Build history of the part. All positions in model axes, mm. A direction names the side the tool comes from. Give positions to 0.01 mm unless a question says otherwise; leave off trailing zeros. Order: outer loops, then holes, each group sorted by start corner. A loop starts at its lowest first (then second) coordinate and runs counter-clockwise, first axis right, second up. Notation, with made-up numbers: (56, 83.25) - (107, 83.25) arc R38 ccw to (107, 122.25) - close; hole circle Ø5 at (-36.5, 85). An arc over 180 degrees is marked (long way). Use a Markdown table: item, result.
from build123d import *

# Parameters (mm, degrees)
BASE_PLATE_DEPTH                        = 4.7625
OUTSIDEBOSS_DEPTH                       = 50.8
TOPPLATE_MOUNTINGHOLE_8_0_199_DIAMETE_D = 5.1054
PCB_PLATE_DEPTH                         = 12.7
F_4_CLEARANCE_HOLE1_D                   = 3.2639
F_4_CLEARANCE_HOLE1_DEPTH               = 16.002
F_4_CLEARANCE_HOLE1_TIP                 = 0.980574487
SKETCH11_W                              = 87.3125
SKETCH11_H                              = 50.8
SKETCH11_W_2                            = 6.35
SKETCH11_H_2                            = 6.35
CUT_EXTRUDE2_DEPTH                      = 4.7625
SKETCH12_W                              = 78.3336
SKETCH12_H                              = 18.0086
SKETCH12_W_2                            = 76.2
SKETCH12_H_2                            = 15.875
BATTERYHOLDER_DEPTH                     = 44.45
BATTERYLEADFEADER_REACH                 = 128.453
BATTERYLEADFILLETS_R                    = 3.175
CUT_EXTRUDE3_REACH                      = 149.637


with BuildPart() as part:
    # Sketch1 → Base_Plate (new body)
    with BuildSketch(Plane(origin=(0, 0, 0), x_dir=(1, 0, 0), z_dir=(0, 1, 0))):
        with BuildLine():
            Line((-53.975, 50.8), (53.975, 50.8))
            ThreePointArc((53.975, 50.8), (60.710192091, 48.010192091), (63.5, 41.275))
            Line((63.5, 41.275), (63.5, -41.275))
            ThreePointArc((63.5, -41.275), (60.710192091, -48.010192091), (53.975, -50.8))
            Line((53.975, -50.8), (-53.975, -50.8))
            ThreePointArc((-53.975, -50.8), (-60.710192091, -48.010192091), (-63.5, -41.275))
            Line((-63.5, -41.275), (-63.5, 41.275))
            ThreePointArc((-63.5, 41.275), (-60.710192091, 48.010192091), (-53.975, 50.8))
        make_face()
    extrude(amount=BASE_PLATE_DEPTH)

    # Sketch2 → OutsideBoss (add)
    with BuildSketch(Plane(origin=(0, 4.7625, 0), x_dir=(1, 0, 0), z_dir=(0, 1, 0))):
        with BuildLine():
            Line((-53.975, -50.8), (53.975, -50.8))
            ThreePointArc((53.975, -50.8), (60.710192091, -48.010192091), (63.5, -41.275))
            Line((63.5, -41.275), (63.5, 41.275))
            ThreePointArc((63.5, 41.275), (60.710192091, 48.010192091), (53.975, 50.8))
            Line((53.975, 50.8), (-53.975, 50.8))
            ThreePointArc((-53.975, 50.8), (-60.710192091, 48.010192091), (-63.5, 41.275))
            Line((-63.5, 41.275), (-63.5, -41.275))
            ThreePointArc((-63.5, -41.275), (-60.710192091, -48.010192091), (-53.975, -50.8))
        make_face()
        with BuildLine():
            Line((-56.1975, 41.275), (-56.1975, -41.275))
            ThreePointArc((-56.1975, -41.275), (-55.546544821, -42.846544821), (-53.975, -43.4975))
            Line((-53.975, -43.4975), (53.975, -43.4975))
            ThreePointArc((53.975, -43.4975), (55.546544821, -42.846544821), (56.1975, -41.275))
            Line((56.1975, -41.275), (56.1975, 41.275))
            ThreePointArc((56.1975, 41.275), (55.546544821, 42.846544821), (53.975, 43.4975))
            Line((53.975, 43.4975), (-53.975, 43.4975))
            ThreePointArc((-53.975, 43.4975), (-55.546544821, 42.846544821), (-56.1975, 41.275))
        make_face(mode=Mode.SUBTRACT)
    extrude(amount=OUTSIDEBOSS_DEPTH)

    # TopPlate_MountingHole_#8 (0.199) Diameter Hole1 (through all)
    with Locations(Plane(origin=(0, 0, 0), x_dir=(-1, 0, 0), z_dir=(0, -1, 0))):
        with Locations((-58.07075, 45.37075), (58.07075, -45.37075), (-58.07075, -45.37075), (58.07075, 45.37075)):
            Hole(TOPPLATE_MOUNTINGHOLE_8_0_199_DIAMETE_D / 2)

    # Sketch8 → PCB_Plate (add)
    with BuildSketch(Plane(origin=(0, 4.7625, 0), x_dir=(1, 0, 0), z_dir=(0, 1, 0))):
        with BuildLine():
            Line((46.83125, -37.1475), (-46.83125, -37.1475))
            ThreePointArc((-46.83125, -37.1475), (-49.07631403, -36.21756403), (-50.00625, -33.9725))
            Line((-50.00625, -33.9725), (-50.00625, 23.1775))
            ThreePointArc((-50.00625, 23.1775), (-49.07631403, 25.42256403), (-46.83125, 26.3525))
            Line((-46.83125, 26.3525), (46.83125, 26.3525))
            ThreePointArc((46.83125, 26.3525), (49.07631403, 25.42256403), (50.00625, 23.1775))
            Line((50.00625, 23.1775), (50.00625, -33.9725))
            ThreePointArc((50.00625, -33.9725), (49.07631403, -36.21756403), (46.83125, -37.1475))
        make_face()
    extrude(amount=PCB_PLATE_DEPTH)

    # #4 Clearance Hole1
    with Locations(Plane(origin=(0, 17.4625, 0), x_dir=(1, 0, 0), z_dir=(0, 1, 0))):
        with Locations((-46.83125, 23.574375), (46.83125, 23.574375), (-46.83125, -34.369375), (46.83125, -34.369375)):
            Hole(F_4_CLEARANCE_HOLE1_D / 2, depth=F_4_CLEARANCE_HOLE1_DEPTH)
            with Locations((0, 0, -(F_4_CLEARANCE_HOLE1_DEPTH + F_4_CLEARANCE_HOLE1_TIP / 2))):  # 118° drill point
                Cone(0, F_4_CLEARANCE_HOLE1_D / 2, F_4_CLEARANCE_HOLE1_TIP, mode=Mode.SUBTRACT)

    # Sketch11 → Cut-Extrude2 (cut)
    with BuildSketch(Plane(origin=(0, 17.4625, 0), x_dir=(1, 0, 0), z_dir=(0, 1, 0))):
        with Locations((0, -5.3975)):
            Rectangle(SKETCH11_W, SKETCH11_H)
        with Locations((46.83125, -5.3975)):
            Rectangle(SKETCH11_W_2, SKETCH11_H)
        with Locations((0, 23.1775)):
            Rectangle(SKETCH11_W, SKETCH11_H_2)
        with Locations((0, -33.9725)):
            Rectangle(SKETCH11_W, SKETCH11_H_2)
        with Locations((-46.83125, -5.3975)):
            Rectangle(SKETCH11_W_2, SKETCH11_H)
    extrude(amount=-CUT_EXTRUDE2_DEPTH, mode=Mode.SUBTRACT)

    # Sketch12 → BatteryHolder (add)
    with BuildSketch(Plane(origin=(0, 4.7625, 0), x_dir=(1, 0, 0), z_dir=(0, 1, 0))):
        with Locations((0, 35.56)):
            Rectangle(SKETCH12_W, SKETCH12_H)
        with Locations((0, 35.56)):
            Rectangle(SKETCH12_W_2, SKETCH12_H_2, mode=Mode.SUBTRACT)
    extrude(amount=BATTERYHOLDER_DEPTH)

    # Sketch13 → BatteryLeadFeader (cut, up to next)
    with BuildSketch(Plane(origin=(-38.1, 0, 0), x_dir=(0, 0, -1), z_dir=(1, 0, 0)), mode=Mode.PRIVATE) as batteryleadfeader_sk1:
        with BuildLine():
            Line((38.735, 23.8125), (38.735, 49.2125))
            Line((38.735, 49.2125), (32.385, 49.2125))
            Line((32.385, 49.2125), (32.385, 23.8125))
            ThreePointArc((32.385, 23.8125), (35.56, 26.9875), (38.735, 23.8125))
        make_face()
    batteryleadfeader_tool1 = extrude(batteryleadfeader_sk1.sketch, amount=-BATTERYLEADFEADER_REACH, mode=Mode.PRIVATE) & part.part
    # Sketch13 → BatteryLeadFeader (cut, up to next)
    with BuildSketch(Plane(origin=(-38.1, 0, 0), x_dir=(0, 0, -1), z_dir=(1, 0, 0)), mode=Mode.PRIVATE) as batteryleadfeader_sk2:
        with BuildLine():
            ThreePointArc((32.385, 23.8125), (35.56, 20.6375), (38.735, 23.8125))
            Line((38.735, 23.8125), (32.385, 23.8125))
        make_face()
    batteryleadfeader_tool2 = extrude(batteryleadfeader_sk2.sketch, amount=-BATTERYLEADFEADER_REACH, mode=Mode.PRIVATE) & part.part
    # Sketch13 → BatteryLeadFeader (cut, up to next)
    with BuildSketch(Plane(origin=(-38.1, 0, 0), x_dir=(0, 0, -1), z_dir=(1, 0, 0)), mode=Mode.PRIVATE) as batteryleadfeader_sk3:
        with BuildLine():
            Line((32.385, 23.8125), (38.735, 23.8125))
            ThreePointArc((38.735, 23.8125), (35.56, 26.9875), (32.385, 23.8125))
        make_face()
    batteryleadfeader_tool3 = extrude(batteryleadfeader_sk3.sketch, amount=-BATTERYLEADFEADER_REACH, mode=Mode.PRIVATE) & part.part
    # Sketch13 → BatteryLeadFeader (cut, up to next)
    with BuildSketch(Plane(origin=(-38.1, 0, 0), x_dir=(0, 0, -1), z_dir=(1, 0, 0)), mode=Mode.PRIVATE) as batteryleadfeader_sk4:
        with BuildLine():
            ThreePointArc((32.385, 23.8125), (35.56, 20.6375), (38.735, 23.8125))
            Line((38.735, 23.8125), (32.385, 23.8125))
        make_face()
    batteryleadfeader_tool4 = extrude(batteryleadfeader_sk4.sketch, amount=-BATTERYLEADFEADER_REACH, mode=Mode.PRIVATE) & part.part
    # Sketch13 → BatteryLeadFeader (cut, up to next)
    with BuildSketch(Plane(origin=(-38.1, 0, 0), x_dir=(0, 0, -1), z_dir=(1, 0, 0)), mode=Mode.PRIVATE) as batteryleadfeader_sk5:
        with BuildLine():
            Line((32.385, 23.8125), (38.735, 23.8125))
            ThreePointArc((38.735, 23.8125), (35.56, 26.9875), (32.385, 23.8125))
        make_face()
    batteryleadfeader_tool5 = extrude(batteryleadfeader_sk5.sketch, amount=-BATTERYLEADFEADER_REACH, mode=Mode.PRIVATE) & part.part
    add(batteryleadfeader_tool1.solids().sort_by_distance((-38.1, 37.748358, -35.56))[0], mode=Mode.SUBTRACT)
    add(batteryleadfeader_tool2.solids().sort_by_distance((-38.1, 22.464988, -35.56))[0], mode=Mode.SUBTRACT)
    add(batteryleadfeader_tool3.solids().sort_by_distance((-38.1, 25.160012, -35.56))[0], mode=Mode.SUBTRACT)
    add(batteryleadfeader_tool4.solids().sort_by_distance((-38.1, 22.464988, -35.56))[0], mode=Mode.SUBTRACT)
    add(batteryleadfeader_tool5.solids().sort_by_distance((-38.1, 25.160012, -35.56))[0], mode=Mode.SUBTRACT)

    # BatteryLeadFillets
    batteryleadfillets_edges = [part.edges().sort_by_distance(p)[0] for p in [
        (-38.6334, 49.2125, -38.735),
        (-38.6334, 49.2125, -32.385),
    ]]
    fillet(batteryleadfillets_edges, radius=BATTERYLEADFILLETS_R)

    # Sketch14 → Cut-Extrude3 (cut, up to next)
    with BuildSketch(Plane.ZY.offset(63.5), mode=Mode.PRIVATE) as cut_extrude3_sk1:
        with BuildLine():
            Line((-26.3525, 20.6375), (-26.3525, 30.1625))
            ThreePointArc((-26.3525, 30.1625), (-25.42256403, 32.40756403), (-23.1775, 33.3375))
            Line((-23.1775, 33.3375), (33.9725, 33.3375))
            ThreePointArc((33.9725, 33.3375), (36.21756403, 32.40756403), (37.1475, 30.1625))
            Line((37.1475, 30.1625), (37.1475, 20.6375))
            ThreePointArc((37.1475, 20.6375), (36.21756403, 18.39243597), (33.9725, 17.4625))
            Line((33.9725, 17.4625), (-23.1775, 17.4625))
            ThreePointArc((-23.1775, 17.4625), (-25.42256403, 18.39243597), (-26.3525, 20.6375))
        make_face()
    cut_extrude3_tool1 = extrude(cut_extrude3_sk1.sketch, amount=-CUT_EXTRUDE3_REACH, mode=Mode.PRIVATE) & part.part
    add(cut_extrude3_tool1.solids().sort_by_distance((-63.5, 25.4, 5.3975))[0], mode=Mode.SUBTRACT)


solid = part.part
1) Slice it at D-D (y = 39). State how many separate pieces and enclosed holes the cut face has, and give its area (3 significant figures).
Computed:
| item | result |
|---|---|
| separate pieces | 1 |
| enclosed holes | 5 |
| area | 3,080 mm² |
2) Slice it at B-B (x = 25.5). Write the cut outline in (y, z), and give its area (3 significant figures).
Computed:
| item | result |
|---|---|
| outline | (0, -50.8) - (55.56, -50.8) - (55.56, -43.5) - (4.76, -43.5) - (4.76, -27.62) - (49.21, -27.62) - (49.21, -26.56) - (4.76, -26.56) - (4.76, -26.35) - (12.7, -26.35) - (12.7, 37.15) - (4.76, 37.15) - (4.76, 43.5) - (55.56, 43.5) - (55.56, 50.8) - (0, 50.8) - close |
| area | 1,780 mm² |
3) Slice it at C-C (z = -35.56). Write the cut outline in (x, y), and give its area (3 significant figures).
Computed:
| item | result |
|---|---|
| outline | (-63.5, 0) - (63.5, 0) - (63.5, 55.56) - (56.2, 55.56) - (56.2, 4.76) - (39.17, 4.76) - (39.17, 49.21) - (38.1, 49.21) - (38.1, 4.76) - (-38.1, 4.76) - (-38.1, 20.64) - (-39.17, 20.64) - (-39.17, 4.76) - (-56.2, 4.76) - (-56.2, 55.56) - (-63.5, 55.56) - close |
| area | 1,410 mm² |
4) Tool access for faces 4 (the cylindrical face through (60.506, 28.17, -46.138)), 5 (the flat face through (43.656, 15, -23)): list every direction of +Z, -Z, +X, -X, +Y, -Y with a clear straight run to the whole face (end or side of a thin tool).
Computed:
| item | result |
|---|---|
| face 4 | +Y, -Y |
| face 5 | +Y |
5) Wall check: line 1 (Z direction, x = -30.5, y = 19.5); line 2 (X direction, y = 10, z = 29); line 3 (X direction, y = 23.5, z = -37.5). Give the ranges that are in metal, low to high. Write a range as from..to.
Computed:
| item | result |
|---|---|
| line 1 | z = -50.8..-43.5, -27.62..-26.56, 43.5..50.8 |
| line 2 | x = -63.5..-56.2, -50.01..50.01, 56.2..63.5 |
| line 3 | x = -63.5..-56.2, 38.1..39.17, 56.2..63.5 |
6) Pin check, flat tips, straight feed: P1, Ø6, axis at x = -11, z = 19.5, coming from the +Y side; P2, Ø4, axis at x = 46.83, z = -23.57, coming from the +Y side; P3, Ø2, axis at x = -46.83, z = -23.57, coming from the +Y side. Stop position of each tip, or through.
Computed:
| item | result |
|---|---|
| P1 | stops at y = 12.7 |
| P2 | stops at y = 17.46 |
| P3 | stops at y = 1.08 |
7) Two-plate mould, pull along Z, no slides. Class faces 1 (the flat face through (1, 8, 37.148)), 2 (the flat face through (-1, 27, 50.8)), 3 (the flat face through (1, 27, -50.8)): +Z half, -Z half, draft (parallel to the pull), parting line (faces both ways), or undercut.
Computed:
| item | result |
|---|---|
| face 1 | undercut |
| face 2 | +Z half |
| face 3 | -Z half |
8) Slice it at A-A (z = 1.5). Write the cut outline in (x, y).
Computed:
| item | result |
|---|---|
| outline | (-63.5, 0) - (63.5, 0) - (63.5, 55.56) - (56.2, 55.56) - (56.2, 4.76) - (50.01, 4.76) - (50.01, 12.7) - (-50.01, 12.7) - (-50.01, 4.76) - (-56.2, 4.76) - (-56.2, 17.46) - (-63.5, 17.46) - close; (-63.5, 33.34) - (-56.2, 33.34) - (-56.2, 55.56) - (-63.5, 55.56) - close |
